Build history of the part. All positions in model axes, mm. A direction names the side the tool comes from. Give positions to 0.01 mm unless a question says otherwise; leave off trailing zeros. Loops run counter-clockwise (first coordinate to the right, second up) from the corner with the lowest first, then second, coordinate; pieces in that order, holes last. Notation, with made-up numbers: (55, 33) -> (65, 33) arc R10 ccw to (65, 48) -> close; hole circle Ø5 at (-38.75, -40). An arc over 180 degrees is marked (long way). Answer in a Markdown table with one row per item. Add a question column.
from build123d import *

# Parameters (mm, degrees)
SKETCH1_R           = 21.875
BOSS_EXTRUDE1_DEPTH = 13
SKETCH2_R           = 11
CUT_EXTRUDE1_DEPTH  = 7
CUT_EXTRUDE2_REACH  = 33.718
SKETCH3_R           = 8
CUT_EXTRUDE3_REACH  = 35.556
SKETCH4_R           = 1.5
CIRPATTERN1_COUNT   = 6
CHAMFER1_SIZE       = 0.5
SKETCH5_R           = 2.65
CUT_EXTRUDE4_DEPTH  = 1.5
CIRPATTERN2_COUNT   = 6
CUT_EXTRUDE5_DEPTH  = 1.5


with BuildPart() as part:
    # Sketch1 → Boss-Extrude1 (new body)
    with BuildSketch(Plane(origin=(0, 0, 0), x_dir=(1, 0, 0), z_dir=(0, 1, 0))):
        with Locations(Location((0, 0, 0), (0, 0, 90))):
            Circle(SKETCH1_R)
    extrude(amount=BOSS_EXTRUDE1_DEPTH)

    # Sketch2 → Cut-Extrude1 (cut)
    with BuildSketch(Plane(origin=(0, 13, 0), x_dir=(1, 0, 0), z_dir=(0, 1, 0))):
        with Locations(Location((0, 0, 0), (0, 0, 270))):
            Circle(SKETCH2_R)
    extrude(amount=-CUT_EXTRUDE1_DEPTH, mode=Mode.SUBTRACT)

    # Sketch3 → Cut-Extrude2 (cut, up to next)
    with BuildSketch(Plane(origin=(0, 6, 0), x_dir=(1, 0, 0), z_dir=(0, 1, 0)), mode=Mode.PRIVATE) as cut_extrude2_sk1:
        with Locations(Location((0, 0, 0), (0, 0, 270))):
            Circle(SKETCH3_R)
    cut_extrude2_tool1 = extrude(cut_extrude2_sk1.sketch, amount=-CUT_EXTRUDE2_REACH, mode=Mode.PRIVATE) & part.part
    add(cut_extrude2_tool1.solids().sort_by_distance((0, 6, 0))[0], mode=Mode.SUBTRACT)

    # Sketch4 → Cut-Extrude3 (cut, up to next)
    with BuildSketch(Plane(origin=(0, 13, 0), x_dir=(1, 0, 0), z_dir=(0, 1, 0)), mode=Mode.PRIVATE) as cut_extrude3_sk1:
        with Locations(Location((0, 15, 0), (0, 0, 270))):
            Circle(SKETCH4_R)
    cut_extrude3_tool1 = extrude(cut_extrude3_sk1.sketch, amount=-CUT_EXTRUDE3_REACH, mode=Mode.PRIVATE) & part.part
    cut_extrude3 = cut_extrude3_tool1.solids().sort_by_distance((0, 13, -15))[0]
    add(cut_extrude3, mode=Mode.SUBTRACT)

    # CirPattern1: Cut-Extrude3 ×6 about axis
    cirpattern1_axis = Axis((0, 0, 0), (0, 1, 0))
    for i in range(1, CIRPATTERN1_COUNT):
        add(cut_extrude3.rotate(cirpattern1_axis, i * 360 / CIRPATTERN1_COUNT), mode=Mode.SUBTRACT)

    # Chamfer1
    chamfer1_edges = [part.edges().sort_by_distance(p)[0] for p in [
        (0, 6, -8),
        (0, 0, -8),
        (0, 13, -11),
    ]]
    chamfer(chamfer1_edges, length=CHAMFER1_SIZE)

    # Sketch5 → Cut-Extrude4 (cut)
    with BuildSketch(Plane(origin=(0, 13, 0), x_dir=(1, 0, 0), z_dir=(0, 1, 0))):
        with Locations(Location((0, 15, 0), (0, 0, 270))):
            Circle(SKETCH5_R)
    cut_extrude4 = extrude(amount=-CUT_EXTRUDE4_DEPTH, mode=Mode.SUBTRACT)

    # CirPattern2: Cut-Extrude4 ×6 about axis
    cirpattern2_axis = Axis((0, 0, 0), (0, 1, 0))
    for i in range(1, CIRPATTERN2_COUNT):
        add(cut_extrude4.rotate(cirpattern2_axis, i * 360 / CIRPATTERN2_COUNT), mode=Mode.SUBTRACT)

    # Sketch6 → Cut-Extrude5 (cut)
    with BuildSketch(Plane(origin=(0, 0, 0), x_dir=(-1, 0, 0), z_dir=(0, -1, 0))):
        Polygon((14.635829324, 10.35), (11.34493279, 10.35), (9.699484522, 7.5), (11.34493279, 4.65), (14.635829324, 4.65), (16.281277591, 7.5), align=None)
        Polygon((3.290896534, 15), (1.645448267, 17.85), (-1.645448267, 17.85), (-3.290896534, 15), (-1.645448267, 12.15), (1.645448267, 12.15), align=None)
        Polygon((-11.34493279, 10.35), (-14.635829324, 10.35), (-16.281277591, 7.5), (-14.635829324, 4.65), (-11.34493279, 4.65), (-9.699484522, 7.5), align=None)
    cut_extrude5 = extrude(amount=-CUT_EXTRUDE5_DEPTH, mode=Mode.SUBTRACT)

    # Mirror1: Cut-Extrude5 across plane
    add(cut_extrude5.mirror(Plane.XY), mode=Mode.SUBTRACT)


solid = part.part
(1) Saw through at D-D, the plane y = 7.75. List the corners of the cut face in (x, z) (3 decimals), then the cut area to 3 significant figures.
(2) Saw through at B-B, the plane x = 0. State how many separate pieces and enclosed holes the cut face has, then the cut area to 3 significant figures.
(3) Wall check: line 1 along X through (y, z) = (12.4, 7.5); line 2 along X through (y, z) = (7.5, 7.5); line 3 along Z through (x, y) = (-1, 3.25). Give the ranges that are in metal, low to high. Write a range as from..to.
(4) Saw through at A-A, the plane z = 0. List the corners of the cut face in (x, y) (3 decimals).
(5) Flat gauge pins, fed straight in: pin 1 Ø2.5 at (x, z) = (0, 15) entering from +Y; pin 2 Ø1.5 at (x, z) = (-1.5, -16) entering from +Y; pin 3 Ø8 at (x, z) = (-5.5, -1.5) entering from +Y; pin 4 Ø5 at (x, y) = (-7.5, 10.5) entering from -Z. Where does each tip first touch, or does it go through?
(6) Saw through at C-C, the plane x = 12.5. List the corners of the cut face in (y, z).
(7) 3-axis set-ups, long thin cutter, end or side, ignore diameter. For faces 1 (the flat face through (-2, 11.5, -15)), 2 (the cylindrical face through (13, 7, -6)), 3 (the flat face through (2.48, 0.74, -13.595)): which of +Z, -Z, +X, -X, +Y, -Y reach the whole face in a straight line?
(8) Two-plate mould, pull along X, no slides. Class faces 4 (the flat face through (-11, 11.5, -7)), 5 (the flat face through (13, 1, -4.65)), 6 (the cylindrical face through (-21.69, 6.41, 2.85)): released by +X, released by -X, zero draft, split by the parting line, or undercut.
Worked answers:
| question | item | result |
|---|---|---|
| 1 | outline | circle Ø43.75 at (0, 0); hole circle Ø3 at (-12.99, -7.5); hole circle Ø3 at (-12.99, 7.5); hole circle Ø22 at (0, 0); hole circle Ø3 at (0, -15); hole circle Ø3 at (0, 15); hole circle Ø3 at (12.99, -7.5); hole circle Ø3 at (12.99, 7.5) |
| 1 | area | 1,080 mm^2 |
| 2 | separate pieces | 4 |
| 2 | enclosed holes | 0 |
| 2 | area | 225 mm^2 |
| 3 | line 1 | -20.55..-15.64, -10.34..-8.05, 8.05..10.34, 15.64..20.55 |
| 3 | line 2 | -20.55..-14.49, -11.49..-8.05, 8.05..11.49, 14.49..20.55 |
| 3 | line 3 | -21.85..-16.12, -13.88..-7.94, 7.94..13.88, 16.12..21.85 |
| 4 | outline | (-21.875, 0) -> (-8.5, 0) -> (-8, 0.5) -> (-8, 5.5) -> (-8.5, 6) -> (-11, 6) -> (-11, 12.5) -> (-11.5, 13) -> (-21.875, 13) -> close; (8, 0.5) -> (8.5, 0) -> (21.875, 0) -> (21.875, 13) -> (11.5, 13) -> (11, 12.5) -> (11, 6) -> (8.5, 6) -> (8, 5.5) -> close |
| 5 | pin 1 | through |
| 5 | pin 2 | y = 11.5 |
| 5 | pin 3 | y = 6 |
| 5 | pin 4 | z = -21.3 |
| 6 | outline | (0, -17.95) -> (13, -17.95) -> (13, -10.1) -> (11.5, -10.1) -> (11.5, -8.92) -> (1.5, -8.92) -> (1.5, -10.35) -> (0, -10.35) -> close; (0, -4.65) -> (1.5, -4.65) -> (1.5, -6.08) -> (11.5, -6.08) -> (11.5, -4.9) -> (13, -4.9) -> (13, 4.9) -> (11.5, 4.9) -> (11.5, 6.08) -> (1.5, 6.08) -> (1.5, 4.65) -> (0, 4.65) -> close; (0, 10.35) -> (1.5, 10.35) -> (1.5, 8.92) -> (11.5, 8.92) -> (11.5, 10.1) -> (13, 10.1) -> (13, 17.95) -> (0, 17.95) -> close |
| 7 | face 1 | +Y |
| 7 | face 2 | +Y, -Y |
| 7 | face 3 | -Y |
| 8 | face 4 | undercut |
| 8 | face 5 | undercut |
| 8 | face 6 | split by the parting line |
